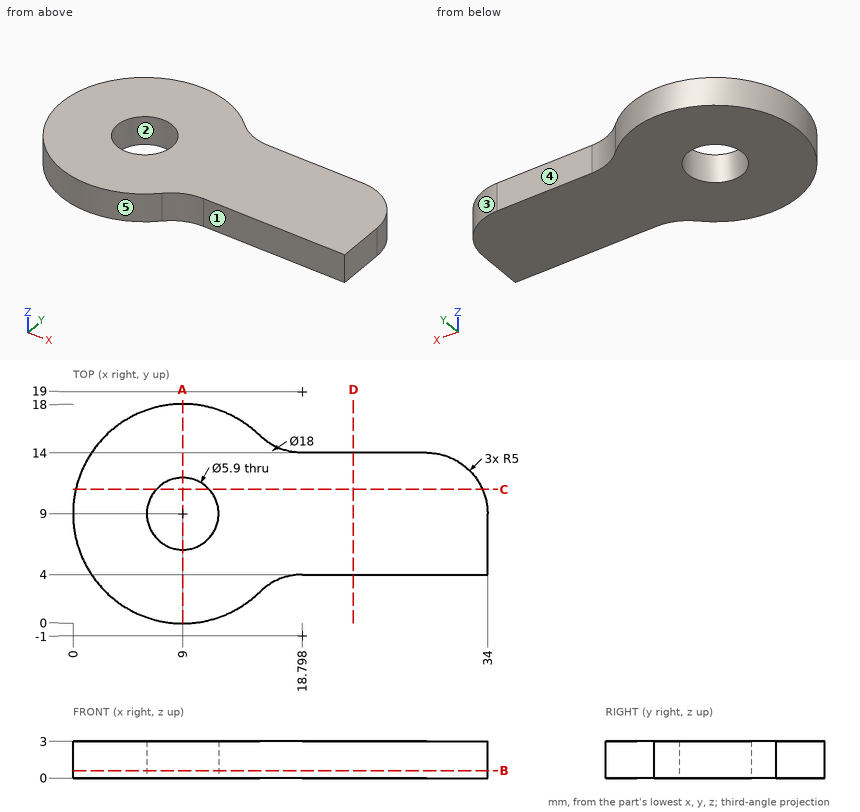
Source: three-view drawing plus pictorial views. Frame: mm from the lowest corner of the part. A direction names the side the tool comes from. Coordinates: 2 decimals unless noted, no trailing zeros. Loops run counter-clockwise (first coordinate to the right, second up) from the corner with the lowest first, then second, coordinate; pieces in that order, holes last. Notation, with made-up numbers: (-23.5, 16.25) -> (21.5, 16.25) arc R27 cw to (21.5, 32.25) -> close; hole circle Ø10 at (11.25, 35.5). An arc over 180 degrees is marked (long way). One line per item, written item: value.
(1) Cut plane D-D (x = 23). Output: boundary loops of the cut face in (y, z), then the cut area to 3 significant figures.
Answer below:
outline: (4, 0) -> (14, 0) -> (14, 3) -> (4, 3) -> close
area: 30.0 mm2
(2) Pin query (flat end, axial travel): pin 1 Ø1.5 at (x, z) = (24.5, 1) entering from -Y; pin 2 Ø1.5 at (x, y) = (10.5, 9) entering from +Z; pin 3 Ø1 at (y, z) = (14, 1.5) entering from -X. Return the tip coordinate at first contact, or that it passes through.
Answer below:
pin 1: stops at y = 4
pin 2: passes through
pin 3: stops at x = 1.21
(3) Ray query, line 1 along X through (y, z) = (9, 1.55); line 2 along X through (y, z) = (7.5, 2.5); line 3 along Y through (x, z) = (27, 2.8). Return the intervals inside material, ascending.
Answer below:
line 1: x = 0 to 6.05, 11.95 to 34
line 2: x = 0.13 to 6.46, 11.54 to 34
line 3: y = 4 to 14
(4) Cut plane A-A (x = 9). Output: boundary loops of the cut face in (y, z), then the cut area to 3 significant figures.
Answer below:
outline: (0, 0) -> (6.05, 0) -> (6.05, 3) -> (0, 3) -> close; (11.95, 0) -> (18, 0) -> (18, 3) -> (11.95, 3) -> close
area: 36.3 mm2
(5) Cut plane C-C (y = 11). Output: boundary loops of the cut face in (x, z) (1 decimal).
Answer below:
outline: (0.2, 0) -> (6.8, 0) -> (6.8, 3) -> (0.2, 3) -> close; (11.2, 0) -> (33.6, 0) -> (33.6, 3) -> (11.2, 3) -> close
(6) Draft query along Y for the marked faces 1, 2 and 3. Return one class per face: pulls with the +Y half, pulls with the -Y half, needs draft (parallel to the pull), parting line crosses it, or undercut.
Answer below:
face 1: pulls with the -Y half
face 2: undercut
face 3: pulls with the +Y half
(7) Cut plane B-B (z = 0.6). Output: boundary loops of the cut face in (x, y).
Answer below:
outline: (15.3, 2.57) arc R5 cw to (18.8, 4) -> (34, 4) -> (34, 9) arc R5 ccw to (29, 14) -> (18.8, 14) arc R5 cw to (15.3, 15.43) arc R9 ccw (long way) to start; hole circle Ø5.9 at (9, 9)
(8) Set-up query: the marked faces 4 and 5. Return all of +Z, -Z, +X, -X, +Y, -Y with unobstructed straight access to the full face (end or side cutting, diameter ignored); none if empty.
Answer below:
face 4: +Z, -Z, +X, +Y
face 5: +Z, -Z
